```python
from build123d import *

# Parameters (mm, degrees)
F1_DEPTH  = 1270
F2_W      = 508
F2_H      = 762
F3_DEPTH  = 1016
F4_W      = 1270
F4_H      = 254
F5_DEPTH  = 1016
F6_W      = 762
F6_H      = 762
F7_DEPTH  = 254.001
F8_W      = 508
F8_H      = 1016
F9_DEPTH  = 254.001
F11_DEPTH = 254.001
F12_W     = 508
F12_H     = 508
F13_DEPTH = 254.001
F14_R     = 254
F15_R     = 253.99999


# Not quite as in the source:
# - a fillet or chamfer is up to 0.001 mm smaller than in the source, because OpenCascade refuses the exact size


with BuildPart() as f1:
    # F0 (on Front) → F1 (new body)
    with BuildSketch(Plane.XZ):
        Polygon((0, 1270), (0, 0), (762, 0), (762, 762), (1524, 762), (1524, 1270), align=None)
    extrude(amount=F1_DEPTH)

    # F2 (on face) → F3 (cut)
    with BuildSketch(Plane.XZ.offset(1270)):
        with Locations((508, 381)):
            Rectangle(F2_W, F2_H)
    extrude(amount=-F3_DEPTH, mode=Mode.SUBTRACT)

    # F4 (on face) → F5 (cut)
    with BuildSketch(Plane.XZ.offset(1270)):
        with Locations((889, 889)):
            Rectangle(F4_W, F4_H)
    extrude(amount=-F5_DEPTH, mode=Mode.SUBTRACT)

    # F6 (on face) → F7 (cut, through all)
    with BuildSketch(Plane(origin=(0, 0, 1016), x_dir=(1, 0, 0), z_dir=(0, 0, -1))):
        with Locations((889, 889)):
            Rectangle(F6_W, F6_H)
    extrude(amount=-F7_DEPTH, mode=Mode.SUBTRACT)

    # F8 (on face) → F9 (cut, through all)
    with BuildSketch(Plane.YZ.offset(254)):
        with Locations((-1016, 508)):
            Rectangle(F8_W, F8_H)
    extrude(amount=-F9_DEPTH, mode=Mode.SUBTRACT)

    # F10 (on face) → F11 (cut, through all)
    with BuildSketch(Plane.YZ.offset(254)):
        Polygon((-254, 0), (-762, 1016), (-762, 0), align=None)
    extrude(amount=-F11_DEPTH, mode=Mode.SUBTRACT)

    # F12 (on face) → F13 (cut, through all)
    with BuildSketch(Plane(origin=(0, 0, 1016), x_dir=(1, 0, 0), z_dir=(0, 0, -1))):
        with Locations((254, 1016)):
            Rectangle(F12_W, F12_H)
    extrude(amount=-F13_DEPTH, mode=Mode.SUBTRACT)

    # F14
    f14_edges = [f1.edges().sort_by_distance(p)[0] for p in [
        (762, -127, 0),
        (1524, -127, 762),
    ]]
    fillet(f14_edges, radius=F14_R)

    # F15 (radius 254 in the source; OpenCascade refuses exactly that, so slightly less here)
    f15_edges = [f1.edges().sort_by_distance(p)[0] for p in [
        (1524, -1270, 1143),
    ]]
    fillet(f15_edges, radius=F15_R)


solid = f1.part
```
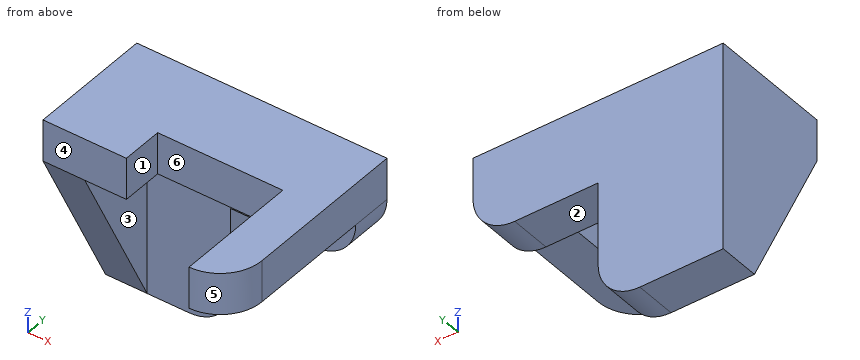
Check sheet for the modelled part. Datum: model origin and axes. Units: mm. Face numbers are marked on the shaded views. A direction names the side the tool comes from. Round coordinates to 2 decimals unless told otherwise and drop trailing zeros. Order: outer loops, then holes, each group sorted by start corner. A loop starts at its lowest first (then second) coordinate and runs counter-clockwise, first axis right, second up. Notation, with made-up numbers: (-3.5, 35.5) -> (30.5, 35.5) arc R7 ccw to (30.5, 41.5) -> close; hole circle Ø7 at (30.25, 4.25). An arc over 180 degrees is marked (long way). Use CSV: the item, a comma, the result in double quotes.
(1) Material ranges on line 1 along Z through (x, y) = (649, -292); line 2 along Y through (x, z) = (512, 290.5); line 3 along X through (y, z) = (-407, 385.5), recorded low to high. Write a range as from..to.
Worked out:
line 1,"1016..1270"
line 2,"-254..0"
line 3,"0..254"
(2) Draft check along X on the marked faces 4, 5 and 6. Enter one of: pulls with the +X half, pulls with the -X half, needs draft (parallel to the pull), parting line crosses it, or undercut.
Worked out:
face 4,"needs draft"
face 5,"pulls with the +X half"
face 6,"undercut"
(3) Tool access check on the marked faces 1, 2 and 3. Record the directions out of +Z, -Z, +X, -X, +Y, -Y that give a thin tool (end or side, any length) a straight path to the whole face; none if there is none.
Worked out:
face 1,"+Z, -Z, -Y"
face 2,"-Z, +X, +Y, -Y"
face 3,"-Z, +X, -Y"
(4) Cross-section at D-D (y = -417.5). Record the boundary of the cut face in (x, z), and give its area (3 significant figures).
Worked out:
outline,"(0, 327) -> (254, 327) -> (254, 1016) -> (1524, 1016) -> (1524, 1270) -> (0, 1270) -> close"
area,"562,000 mm²"
(5) Depth check by flat-ended pin: pin 1 (1.5 mm diameter, centred on y = -1041.5, z = 1087.5, fed in from +X); pin 2 (5 mm diameter, centred on x = 505.5, y = -544, fed in from -Z); pin 3 (10 mm diameter, centred on x = 1051.5, y = -155, fed in from -Z). Enter the tip coordinate at first touch or a pass-through.
Worked out:
pin 1,"x = 1522.79"
pin 2,"z = 1016"
pin 3,"z = 762"
(6) Cross-section at A-A (y = -654). Record the boundary of the cut face in (x, z), and give its area (3 significant figures).
Worked out:
outline,"(0, 800) -> (254, 800) -> (254, 1016) -> (508, 1016) -> (508, 1270) -> (0, 1270) -> close; (1270, 1016) -> (1524, 1016) -> (1524, 1270) -> (1270, 1270) -> close"
area,"248,000 mm²"
(7) Cross-section at C-C (x = 340). Record the boundary of the cut face in (y, z), and give its area (3 significant figures).
Worked out:
outline,"(-762, 1016) -> (-254, 1016) -> (-254, 0) -> (0, 0) -> (0, 1270) -> (-762, 1270) -> close"
area,"452,000 mm²"
